Work out the finished part from the listing and answer in its coordinate system (mm). Round coordinates to 2 decimals unless told otherwise and drop trailing zeros. Order: outer loops, then holes, each group sorted by start corner. A loop starts at its lowest first (then second) coordinate and runs counter-clockwise, first axis right, second up. Notation, with made-up numbers: M 25,77 L 48,77 A27 ccw 48,101 Z; hole C 31.5,77 d7. An arc over 180 degrees is marked long. Return JSON: item names as keys, results as strings.
from build123d import *

# Parameters (mm, degrees)
SKETCH1_R           = 19
BOSS_EXTRUDE1_DEPTH = 2
SKETCH2_R           = 1.6
CUT_EXTRUDE1_DEPTH  = 87.413117357
FILLET1_R           = 10


with BuildPart() as part:
    # Sketch1 → Boss-Extrude1 (new body)
    with BuildSketch(Plane.XY):
        with BuildLine():
            Line((-81.341360029, 18.403724841), (-81.341360029, -18.403724841))
            ThreePointArc((-81.341360029, -18.403724841), (-58.8, -29.1), (-36.258639971, -18.403724841))
            Line((-36.258639971, -18.403724841), (-36.258639971, 18.403724841))
            ThreePointArc((-36.258639971, 18.403724841), (-58.8, 29.1), (-81.341360029, 18.403724841))
        make_face()
        with Locations((-58.8, 0)):
            Circle(SKETCH1_R, mode=Mode.SUBTRACT)
    extrude(amount=BOSS_EXTRUDE1_DEPTH)

    # Sketch2 → Cut-Extrude1 (cut, through all)
    with BuildSketch(Plane.XY.offset(2)):
        with Locations((-58.8, 26)):
            Circle(SKETCH2_R)
        with Locations((-40.415223689, 18.384776311)):
            Circle(SKETCH2_R)
        with Locations((-40.415223689, -18.384776311)):
            Circle(SKETCH2_R)
        with Locations((-58.8, -26)):
            Circle(SKETCH2_R)
        with Locations((-77.184776311, -18.384776311)):
            Circle(SKETCH2_R)
        with Locations((-77.184776311, 18.384776311)):
            Circle(SKETCH2_R)
    extrude(amount=-CUT_EXTRUDE1_DEPTH, mode=Mode.SUBTRACT)

    # Fillet1
    fillet1_edges = [part.edges().sort_by_distance(p)[0] for p in [
        (-81.341360029, -18.403724841, 1),
        (-81.341360029, 18.403724841, 1),
        (-36.258639971, 18.403724841, 1),
        (-36.258639971, -18.403724841, 1),
    ]]
    fillet(fillet1_edges, radius=FILLET1_R)


solid = part.part
Item 1: The mould has two halves that part along Y. Classify faces 1 (the flat face through (-81.341, 0, 1)), 2 (the cylindrical face through (-41.59, -17.3, 1.01)), 3 (the cylindrical face through (-60.4, 26.07, 1.01)), 4 (the cylindrical face through (-58.5, 29.1, 1)): pulls with the +Y half, pulls with the -Y half, needs draft (parallel to the pull), parting line crosses it, or undercut.
Output:
{"face 1": "needs draft", "face 2": "undercut", "face 3": "undercut", "face 4": "pulls with the +Y half"}
Item 2: Each of these flat-tipped pins is pushed along its axis until it touches: pin 1 (6 mm diameter, centred on x = -54.5, y = 21.5, fed in from -Z); pin 2 (3 mm diameter, centred on x = -40.42, y = -18.38, fed in from +Z). Where does it stop, or does it pass through?
Output:
{"pin 1": "stops at z = 0", "pin 2": "passes through"}
Item 3: Consider line 1 along Y through (x, z) = (-58.8, 1.15); line 2 along X through (y, z) = (-0.5, 1.6); line 3 along X through (y, z) = (-8, 0.95). Determine where each line is inside the solid, lowest interval first. Write a range as [from, to].
Output:
{"line 1": "y = [-29.1, -27.6], [-24.4, -19], [19, 24.4], [27.6, 29.1]", "line 2": "x = [-81.34, -77.79], [-39.81, -36.26]", "line 3": "x = [-81.34, -76.03], [-41.57, -36.26]"}
Item 4: Find section B-B (x = -58.8). Determine the outline of the cut face in (y, z).
Output:
{"outline": "M -29.1,0 L -27.6,0 L -27.6,2 L -29.1,2 Z; M -24.4,0 L -19,0 L -19,2 L -24.4,2 Z; M 19,0 L 24.4,0 L 24.4,2 L 19,2 Z; M 27.6,0 L 29.1,0 L 29.1,2 L 27.6,2 Z"}
Item 5: Find section D-D (z = 1.5). Determine the outline of the cut face in (x, y), plus the area to 3 significant figures.
Output:
{"outline": "M -81.34,-14.41 A10 ccw -77.91,-21.95 A29.1 ccw -39.69,-21.95 A10 ccw -36.26,-14.41 L -36.26,14.41 A10 ccw -39.69,21.95 A29.1 ccw -77.91,21.95 A10 ccw -81.34,14.41 Z; hole C -77.18,-18.38 d3.2; hole C -77.18,18.38 d3.2; hole C -58.8,0 d38; hole C -58.8,-26 d3.2; hole C -58.8,26 d3.2; hole C -40.42,-18.38 d3.2; hole C -40.42,18.38 d3.2", "area": "1,140 mm^2"}
Item 6: Find section A-A (y = 0). Determine the outline of the cut face in (x, z), plus the area to 3 significant figures.
Output:
{"outline": "M -81.34,0 L -77.8,0 L -77.8,2 L -81.34,2 Z; M -39.8,0 L -36.26,0 L -36.26,2 L -39.8,2 Z", "area": "14.2 mm^2"}
Item 7: Find section C-C (x = -73). Determine the outline of the cut face in (y, z).
Output:
{"outline": "M -25.4,0 L -12.62,0 L -12.62,2 L -25.4,2 Z; M 12.62,0 L 25.4,0 L 25.4,2 L 12.62,2 Z"}
